Verification items for the finished model (mm, model axes). A direction names the side the tool comes from. Coordinates: 2 decimals unless noted, no trailing zeros. Loops run counter-clockwise (first coordinate to the right, second up) from the corner with the lowest first, then second, coordinate; pieces in that order, holes last. Notation, with made-up numbers: (0.5, -19) - (26.5, -19) arc R11 ccw to (26.5, -14) - close; hole circle Ø6 at (3, -31). An arc over 180 degrees is marked (long way). Answer as CSV lines item,"result". Start each with the question number.
1. Gauge pin test, flat ends, axial feed: P1, Ø5, axis at x = 0, y = 7.5, coming from the -Z side; P2, Ø6, axis at x = -20.5, y = 8.5, coming from the +Z side; P3, Ø12, axis at x = 2.5, y = 10.5, coming from the +Z side. Record the tip position at first contact, or that the pin passes through.
2. Material ranges on line 1 (X direction, y = -0.5, z = 14.5); line 2 (Y direction, x = -18.5, z = 37.5); line 3 (Z direction, x = -29, y = 2.5), recorded low to high. Write a range as [from, to].
3. Release check for a two-part mould opening along X. For faces 1 (the cylindrical face through (-4.92, -13.85, 8.64)), 2 (the flat face through (-34.601, -8, 39)), 3 (the cylindrical face through (-25.209, 3.243, 41.793)), 4 (the flat face through (7.34, 1.65, 19.05)) record: pulls with the +X half, pulls with the -X half, needs draft (parallel to the pull), parting line crosses it, or undercut.
4. Set-up check for faces 5 (the flat face through (1, -10.3, 0)), 6 (the cylindrical face through (7.68, 0.47, 9.39)), 7 (the flat face through (-15.551, 2.4, 41.8)): record each of +Z, -Z, +X, -X, +Y, -Y from which the full face is reachable in a straight line by a thin tool's end or side.
5. Cross-section at A-A (z = 13.5). Enter the section's corners in (x, y) (3 decimals), plus the area to 3 significant figures.
Autodesk Inventor part; units mm, degrees
ref_plane "YZ Plane" through (0, 0, 0) normal (1, 0, 0) x (0, 1, 0)
ref_plane "XZ Plane" through (0, 0, 0) normal (0, 1, 0) x (-1, 0, 0)
ref_plane "XY Plane" through (0, 0, 0) normal (0, 0, 1) x (1, 0, 0)
sketch "Sketch1" plane through (0, 0, 0) normal (0, 0, 1) x (1, 0, 0)
  circle A0 centre (-3.105, 0) radius 13.97
  circle A1 centre (-3.105, 0) radius 10.414
  point P0 (0, 0)
  dimension "d0" = 27.94
  dimension "d2" = 20.828
extrude "Extrusion1" add sketch "Sketch1" along normal blind 17.526
sketch "Sketch2" plane through (-3.105, 0, 17.526) normal (0, 0, 1) x (1, 0, 0)
  circle A0 centre (0, 0) radius 10.414
  circle A1 centre (0, 0) radius 13.97
  line L0 (-13.97, 13.97) -> (-13.97, -13.97)
  line L1 (-13.97, -13.97) -> (13.97, -13.97)
  point P0 (3.105, 0)
revolve "Revolution1" add sketch "Sketch2" angle 90 about axis through (-17.075, 13.97, 17.526) along (0, -1, 0) contours A1
sketch "Sketch3" plane through (-17.075, 0, 31.496) normal (-1, 0, 0) x (0, 0, 1)
  circle A0 centre (0, 0) radius 10.414
  circle A1 centre (0, 0) radius 13.97
  point P0 (-13.97, 0)
  point P1 (-31.496, 0)
extrude "Extrusion2" add sketch "Sketch3" along normal blind 17.526
sketch "Sketch4" plane through (-34.601, 0, 31.496) normal (-1, 0, 0) x (0, 0, 1)
  circle A0 centre (0, 0) radius 10.414
  circle A1 centre (0, 0) radius 13.97
  circle A2 centre (0, 0) radius 10.795
  point P0 (-31.496, 0)
  dimension "d8" = 21.59
extrude "Extrusion3" cut sketch "Sketch4" against normal blind 19.05 contours A2
sketch "Sketch5" plane through (-3.105, 0, 0) normal (0, 0, -1) x (-1, 0, 0)
  circle A0 centre (0, 0) radius 10.414
  circle A1 centre (0, 0) radius 13.97
  circle A2 centre (0, 0) radius 10.795
  point P0 (-3.105, 0)
  dimension "d12" = 21.59
extrude "Extrusion4" cut sketch "Sketch5" against normal blind 19.05 contours A2
properties part number "0.5 Elbow" material "PVC-Piping"
Values follow:
1,P1,"stops at z = 17.53"
1,P2,"stops at z = 44.34"
1,P3,"stops at z = 39.1"
2,line 1,"x = [-17.07, -13.89], [7.68, 10.86]"
2,line 2,"y = [-12.61, -8.97], [8.97, 12.61]"
2,line 3,"z = [17.75, 20.99], [42, 45.24]"
3,face 1,"parting line crosses it"
3,face 2,"pulls with the -X half"
3,face 3,"needs draft"
3,face 4,"undercut"
4,face 5,"-Z, +X, -X, +Y, -Y"
4,face 6,"-Z"
4,face 7,"-X"
5,outline,"circle Ø27.94 at (-3.105, 0); hole circle Ø21.59 at (-3.105, 0)"
5,area,"247 mm²"
